from build123d import *

# Parameters (mm, degrees)
F0_W        = 100
F0_H        = 170
F1_DEPTH    = 40
F2_R        = 39.99999
F3_W        = 100
F3_H        = 59.416816481
F4_DEPTH    = 25
F5_T1_DEPTH = 285.4049621774
F7_DEPTH    = 25
F8_W        = 93.7445983291
F8_H        = 163.0899235606
F9_DEPTH    = 25
F11_DEPTH   = 25
F12_W       = 79.9397490919
F12_H       = 50.4037756473
F13_DEPTH   = 10


# Not quite as in the source:
# - a fillet or chamfer that OpenCascade refuses, or shapes differently, is made with other operations: its cross-section is extruded or revolved along the edge and cut away or added
# - a fillet or chamfer is up to 0.001 mm smaller than in the source, because OpenCascade refuses the exact size


with BuildPart() as f1:
    # F0 (on Top) → F1 (new body)
    with BuildSketch(Plane.XY):
        with Locations((0, 3.7849953254)):
            Rectangle(F0_W, F0_H)
    extrude(amount=F1_DEPTH)

    # F2 (radius 40 in the source; OpenCascade refuses exactly that, so slightly less here)
    f2_edges = [f1.edges().sort_by_distance(p)[0] for p in [
        (0, 88.784995, 40),
    ]]
    fillet(f2_edges, radius=F2_R)

    # F3 (on face) → F4 (join)
    with BuildSketch(Plane.XY.offset(40)):
        with Locations((0, 19.0765870849)):
            Rectangle(F3_W, F3_H)
    extrude(amount=F4_DEPTH)

    # F5: fillet of radius 40 on 1 edges, made by hand

    # F5_s2 → F5_t1 (cut)
    with BuildSketch(Plane.YZ.offset(-142.7024810887)):
        with BuildLine():
            ThreePointArc((48.7849953254, 40), (34.0646826649, 58.1662479036), (11.7040028899, 65))
            Line((11.7040028899, 65), (48.7849953254, 65))
            Line((48.7849953254, 65), (48.7849953254, 40))
        make_face()
    extrude(amount=F5_T1_DEPTH, mode=Mode.SUBTRACT)

    # F6 (on face) → F7 (cut)
    with BuildSketch(Plane.YZ.offset(50)):
        with BuildLine():
            Line((-74.4276870787, 0), (-34.4276870787, 0))
            ThreePointArc((-34.4276870787, 0), (-54.4276870787, 20), (-74.4276870787, 0))
        make_face()
        with BuildLine():
            ThreePointArc((80.5723129213, 0), (60.5723129213, 20), (40.5723129213, 0))
            Line((40.5723129213, 0), (80.5723129213, 0))
        make_face()
    extrude(amount=-F7_DEPTH, mode=Mode.SUBTRACT)

    # F8 (on face) → F9 (cut)
    with BuildSketch(Plane(origin=(0, 0, 0), x_dir=(1, 0, 0), z_dir=(0, 0, -1))):
        with Locations((-0.160522759, -3.6244727671)):
            Rectangle(F8_W, F8_H)
    extrude(amount=-F9_DEPTH, mode=Mode.SUBTRACT)

    # F10 (on face) → F11 (cut)
    with BuildSketch(Plane(origin=(-50, 0, 0), x_dir=(0, -1, 0), z_dir=(-1, 0, 0))):
        with BuildLine():
            ThreePointArc((-77.0112355053, 0), (-57.0112355053, -20), (-37.0112355053, 0))
            Line((-37.0112355053, 0), (-77.0112355053, 0))
        make_face()
        with BuildLine():
            ThreePointArc((77.9887644947, 0), (57.9887644947, 20), (37.9887644947, 0))
            Line((37.9887644947, 0), (77.9887644947, 0))
        make_face()
        with BuildLine():
            Line((-77.0112355053, 0), (-37.0112355053, 0))
            ThreePointArc((-37.0112355053, 0), (-57.0112355053, 20), (-77.0112355053, 0))
        make_face()
        with BuildLine():
            Line((77.9887644947, 0), (37.9887644947, 0))
            ThreePointArc((37.9887644947, 0), (57.9887644947, -20), (77.9887644947, 0))
        make_face()
    extrude(amount=-F11_DEPTH, mode=Mode.SUBTRACT)

    # F12 (on face) → F13 (cut)
    with BuildSketch(Plane.XY.offset(40)):
        with Locations((-1.6052145511, -47.2608646378)):
            Rectangle(F12_W, F12_H)
    extrude(amount=-F13_DEPTH, mode=Mode.SUBTRACT)


solid = f1.part
Could you check a few things on this model? Use its own coordinates, in mm. A direction names the side the tool comes from. Coordinates: 2 decimals unless noted, no trailing zeros. Write each loop counter-clockwise with the first axis right and the second up, starting at its lowest first coordinate (ties: lowest second). Pieces come first, ordered by that corner, then holes. Notation, with made-up numbers: M -18,27.25 L 32,27.25 A19 ccw 32,44.25 Z; hole C 58.5,-31.5 d3. An arc over 180 degrees is marked long. One line per question, with ' | ' between items.
1) Imagine slicing it at B-B, the plane z = 32. Write out the boundary of the cut face in (x, y) (3 decimals), and give its area (3 significant figures).
Checks:
outline: M -50,-81.215 L 50,-81.215 L 50,72.785 L -50,72.785 Z; hole M -41.575,-72.463 L 38.365,-72.463 L 38.365,-22.059 L -41.575,-22.059 Z | area: 11,400 mm²
2) I need wall thicknesses on probe 1 along X at (y, z) = (75.5, 22); probe 2 along Z at (x, y) = (-21.5, -58); probe 3 along Z at (x, y) = (44.5, -11). Which ranges of each line are inside material? Lowest first, please. Write a range as [from, to].
Checks:
probe 1: [-50, -47.03], [46.71, 50] | probe 2: [25, 30] | probe 3: [25, 40]
3) Imagine slicing it at C-C, the plane y = 53. Write out the boundary of the cut face in (x, z).
Checks:
outline: M -50,19.59 L -47.03,19.59 L -47.03,25 L 46.71,25 L 46.71,18.51 L 50,18.51 L 50,39.78 L -50,39.78 Z
4) Imagine slicing it at D-D, the plane z = 11. Write out the boundary of the cut face in (x, y) (3 decimals).
Checks:
outline: M -50,-81.215 L 50,-81.215 L 50,-71.131 L 46.712,-71.131 L 46.712,-77.92 L -47.033,-77.92 L -47.033,-74.692 L -50,-74.692 Z; M -50,-41.285 L -47.033,-41.285 L -47.033,40.308 L -50,40.308 Z; M -50,73.715 L -47.033,73.715 L -47.033,85.169 L 46.712,85.169 L 46.712,77.276 L 50,77.276 L 50,87.243 L -50,87.243 Z; M 46.712,-37.724 L 50,-37.724 L 50,43.869 L 46.712,43.869 Z
5) For pin 1 Ø15 at (x, y) = (-9, -48.5) entering from +Z; pin 2 Ø5 at (x, z) = (-12, 37) entering from +Y; pin 3 Ø1.5 at (x, z) = (-33, 45) entering from -Y, each with a flat end and sliding along its axis, tell me the tip position at first contact or that it passes through.
Checks:
pin 1: z = 30 | pin 2: y = 69.03 | pin 3: y = -10.63
6) If we mould it in two halves opening along Y, with no side actions, what happens to faces 1 (the face through (48.379, -53.988, 19.995)), 2 (the face through (0.7, 77.38, 27.97)), 3 (the face through (-1, 1, 65)), 4 (the face through (-1, -77.92, 12))? For each: released by +Y, released by -Y, zero draft, split by the parting line, or undercut.
Checks:
face 1: undercut | face 2: released by +Y | face 3: zero draft | face 4: undercut
7) For faces 5 (the face through (-49, 57, 20)), 6 (the face through (-1, 0, 25)), 7 (the face through (-1, -10.632, 52)), which set-ups out of +Z, -Z, +X, -X, +Y, -Y let a thin tool reach every point of the face, with its end or its side?
Checks:
face 5: -Z, -X | face 6: -Z, +Y | face 7: +Z, +X, -X, -Y
